```python
from build123d import *

# Parameters (mm, degrees)
SKETCH1_W           = 86
SKETCH1_H           = 80
BOSS_EXTRUDE1_DEPTH = 3
SKETCH2_W           = 3
SKETCH2_H           = 80
BOSS_EXTRUDE2_DEPTH = 120
SKETCH3_R           = 16
CUT_EXTRUDE1_DEPTH  = 120
SKETCH4_R           = 2.5
CUT_EXTRUDE2_DEPTH  = 120
SKETCH5_R           = 5
CUT_EXTRUDE3_DEPTH  = 156.32224567


with BuildPart() as part:
    # Sketch1 → Boss-Extrude1 (new body)
    with BuildSketch(Plane.XY):
        Rectangle(SKETCH1_W, SKETCH1_H)
    extrude(amount=BOSS_EXTRUDE1_DEPTH)

    # Sketch2 → Boss-Extrude2 (add)
    with BuildSketch(Plane.XY.offset(3)):
        with Locations((-41.5, 0)):
            Rectangle(SKETCH2_W, SKETCH2_H)
        with Locations((41.5, 0)):
            Rectangle(SKETCH2_W, SKETCH2_H)
    extrude(amount=BOSS_EXTRUDE2_DEPTH)

    # Sketch3 → Cut-Extrude1 (cut)
    with BuildSketch(Plane(origin=(0, 0, 0), x_dir=(-1, 0, 0), z_dir=(0, 0, -1))):
        with Locations((15, 0)):
            Circle(SKETCH3_R)
    extrude(amount=-CUT_EXTRUDE1_DEPTH, mode=Mode.SUBTRACT)

    # Sketch4 → Cut-Extrude2 (cut)
    with BuildSketch(Plane(origin=(0, 0, 0), x_dir=(-1, 0, 0), z_dir=(0, 0, -1))):
        with Locations((-33.23, 33.23)):
            Circle(SKETCH4_R)
        with Locations((-33.23, -33.23)):
            Circle(SKETCH4_R)
        with Locations((33.23, -33.23)):
            Circle(SKETCH4_R)
        with Locations((33.23, 33.23)):
            Circle(SKETCH4_R)
    extrude(amount=-CUT_EXTRUDE2_DEPTH, mode=Mode.SUBTRACT)

    # Sketch5 → Cut-Extrude3 (cut, through all)
    with BuildSketch(Plane(origin=(43, 0, 0), x_dir=(0, 0, -1), z_dir=(1, 0, 0))):
        with Locations(Location((-50, 20, 0), (0, 0, 90))):
            Circle(SKETCH5_R)
        with Locations(Location((-50, -20, 0), (0, 0, 90))):
            Circle(SKETCH5_R)
        with Locations(Location((-70, 20, 0), (0, 0, 90))):
            Circle(SKETCH5_R)
        with Locations(Location((-70, -20, 0), (0, 0, 90))):
            Circle(SKETCH5_R)
    extrude(amount=-CUT_EXTRUDE3_DEPTH, mode=Mode.SUBTRACT)


solid = part.part
```
Part model, mm, in its own coordinate system. A direction names the side the tool comes from. Round coordinates to 2 decimals unless told otherwise and drop trailing zeros. Write each loop counter-clockwise with the first axis right and the second up, starting at its lowest first coordinate (ties: lowest second). Pieces come first, ordered by that corner, then holes. Notation, with made-up numbers: M 7,7.5 L 25,7.5 A23 ccw 25,34.5 Z; hole C -16,62.25 d11. An arc over 180 degrees is marked long. Answer as CSV lines item,"result". Start each with the question number.
1) Band-saw the part on A-A (z = 70). List the corners of the cut face in (x, y), then the cut area to 3 significant figures.
2) Band-saw the part on C-C (y = 20). List the corners of the cut face in (x, z).
3) Mould opens along Y. For faces 1 (the face through (-11.53, -15.62, 1.48)), 2 (the face through (40, -1, 62)), 3 (the face through (0, 40, 2)), 4 (the face through (0, -40, 2)) say: +Y half, -Y half, draft (parallel to the pull), parting line (faces both ways), or undercut.
4) Band-saw the part on D-D (z = 96). List the corners of the cut face in (x, y).
5) Drop flat-ended pins along their axis: pin 1 (3 mm diameter, centred on x = 33.23, y = -33.23, fed in from +Z); pin 2 (8 mm diameter, centred on x = -33.23, y = 33.23, fed in from -Z); pin 3 (5 mm diameter, centred on x = -34, y = -7.5, fed in from +Z). Give the stop position or say it passes through.
6) Band-saw the part on B-B (x = 33.23). List the corners of the cut face in (y, z), then the cut area to 3 significant figures.
7) Which spindle directions (+Z, -Z, +X, -X, +Y, -Y) get a long thin tool onto all of the face, cutting with end or side? Do faces 5 (the face through (-32.69, 30.79, 1.48)), 6 (the face through (-40, -1, 62)). Say none if no direction does.
8) Drill centre lines: L1, parallel to Y at x = 33.23, z = 0.9; L2, parallel to Z at x = 42.25, y = 20; L3, parallel to X at y = -29, z = 110. Where is each one in solid material? Low to high.
Worked out:
1,outline,"M -43,-40 L -40,-40 L -40,-25 L -43,-25 Z; M -43,-15 L -40,-15 L -40,15 L -43,15 Z; M -43,25 L -40,25 L -40,40 L -43,40 Z; M 40,-40 L 43,-40 L 43,-25 L 40,-25 Z; M 40,-15 L 43,-15 L 43,15 L 40,15 Z; M 40,25 L 43,25 L 43,40 L 40,40 Z"
1,area,"360 mm²"
2,outline,"M -43,0 L 43,0 L 43,45 L 40,45 L 40,3 L -40,3 L -40,45 L -43,45 Z; M -43,55 L -40,55 L -40,65 L -43,65 Z; M -43,75 L -40,75 L -40,123 L -43,123 Z; M 40,55 L 43,55 L 43,65 L 40,65 Z; M 40,75 L 43,75 L 43,123 L 40,123 Z"
3,face 1,"undercut"
3,face 2,"draft"
3,face 3,"+Y half"
3,face 4,"-Y half"
4,outline,"M -43,-40 L -40,-40 L -40,40 L -43,40 Z; M 40,-40 L 43,-40 L 43,40 L 40,40 Z"
5,pin 1,"through"
5,pin 2,"z = 0"
5,pin 3,"z = 3"
6,outline,"M -40,0 L -35.73,0 L -35.73,3 L -40,3 Z; M -30.73,0 L 30.73,0 L 30.73,3 L -30.73,3 Z; M 35.73,0 L 40,0 L 40,3 L 35.73,3 Z"
6,area,"210 mm²"
7,face 5,"+Z, -Z"
7,face 6,"+Z, +Y, -Y"
8,L1,"-40 to -35.73, -30.73 to 30.73, 35.73 to 40"
8,L2,"0 to 45, 55 to 65, 75 to 123"
8,L3,"-43 to -40, 40 to 43"
